from build123d import *

# Parameters (mm, degrees)
F1_DEPTH = 25
F2_R     = 2.296991
F2_R_2   = 2.582396
F3_DEPTH = 25
F5_DEPTH = 25


with BuildPart() as f1:
    # F0 (on Front) → F1 (new body)
    with BuildSketch(Plane.XZ):
        Polygon((0, 0), (0, 30), (-1.5, 30), (-1.5, 1.5), (-30, 1.5), (-30, 0), align=None)
    extrude(amount=F1_DEPTH)

    # F2 (on face) → F3 (cut)
    with BuildSketch(Plane.XY.offset(1.5)):
        with Locations((-22, -17)):
            Circle(F2_R)
        with Locations((-8, -8)):
            Circle(F2_R_2)
    extrude(amount=-F3_DEPTH, mode=Mode.SUBTRACT)

    # F4 (on face) → F5 (cut)
    with BuildSketch(Plane.YZ):
        with BuildLine():
            Line((-10.000746, 22.061086), (-10.00074, 21.93918))
            ThreePointArc((-10.00074, 21.93918), (-10, 22.000133), (-10.000746, 22.061086))
        make_face()
        with BuildLine():
            Line((-10, 8.000133), (-10.00074, 21.93918))
            Line((-10.00074, 21.93918), (-10.000746, 22.061086))
            ThreePointArc((-10.000746, 22.061086), (-12.495314, 24.499996), (-14.999007, 22.070455))
            Line((-14.999007, 22.070455), (-14.999007, 21.929545))
            Line((-14.999007, 21.929545), (-14.999007, 8.070455))
            Line((-14.999007, 8.070455), (-14.999007, 7.929545))
            ThreePointArc((-14.999007, 7.929545), (-12.464703, 5.500249), (-10, 8.000133))
        make_face()
        with BuildLine():
            Line((-14.999007, 21.929545), (-14.999007, 22.070455))
            ThreePointArc((-14.999007, 22.070455), (-15, 22), (-14.999007, 21.929545))
        make_face()
        with BuildLine():
            ThreePointArc((-14.999007, 8.070455), (-15, 8), (-14.999007, 7.929545))
            Line((-14.999007, 7.929545), (-14.999007, 8.070455))
        make_face()
    extrude(amount=-F5_DEPTH, mode=Mode.SUBTRACT)


solid = f1.part
Read the model definition and answer for the solid it produces. Units are mm, in the model's axes. A direction names the side the tool comes from. Round coordinates to 2 decimals unless told otherwise and drop trailing zeros. Write each loop counter-clockwise with the first axis right and the second up, starting at its lowest first coordinate (ties: lowest second). Pieces come first, ordered by that corner, then holes.
Q1. Find section A-A on x = -22. Determine the outline of the cut face in (y, z).
Values:
outline: (-25, 0) - (-19.3, 0) - (-19.3, 1.5) - (-25, 1.5) - close; (-14.7, 0) - (0, 0) - (0, 1.5) - (-14.7, 1.5) - close
Q2. Flat-ended cylindrical pins translate along their axes: P1, Ø12.5, axis at y = -11, z = 10, coming from the -X side; P2, Ø7.5, axis at x = -22, y = -17, coming from the +Z side. Find the tip coordinate at first contact, or state that the pin passes through.
Values:
P1: stops at x = -1.5
P2: stops at z = 1.5
Q3. Find section C-C on y = -18.5. Determine the outline of the cut face in (x, z).
Values:
outline: (-30, 0) - (-23.74, 0) - (-23.74, 1.5) - (-30, 1.5) - close; (-20.26, 0) - (0, 0) - (0, 30) - (-1.5, 30) - (-1.5, 1.5) - (-20.26, 1.5) - close
Q4. Find section D-D on y = -12.5. Determine the outline of the cut face in (x, z).
Values:
outline: (-30, 0) - (0, 0) - (0, 5.5) - (-1.5, 5.5) - (-1.5, 1.5) - (-30, 1.5) - close; (-1.5, 24.5) - (0, 24.5) - (0, 30) - (-1.5, 30) - close
Q5. Find section B-B on z = 6. Determine the outline of the cut face in (x, y), and give its area (3 significant figures).
Values:
outline: (-1.5, -25) - (0, -25) - (0, -14) - (-1.5, -14) - close; (-1.5, -11) - (0, -11) - (0, 0) - (-1.5, 0) - close
area: 33.0 mm2
Q6. The mould has two halves that part along Z. Classify faces 4 (the face through (-1, -12, 30)), 5 (the face through (-15, -12, 0)), 6 (the face through (-0.7, -12.4, 24.5)), 7 (the face through (-24.295, -16.899, 0.76)): released by +Z, released by -Z, zero draft, split by the parting line, or undercut.
Values:
face 4: released by +Z
face 5: released by -Z
face 6: undercut
face 7: zero draft
Q7. Straight lines are drawn through the part: line 1 (Y direction, x = -8, z = 0.6); line 2 (Y direction, x = -22, z = 0.7); line 3 (X direction, y = -19.5, z = 4.25). For each, find the intervals that lie inside material, in ascending order.
Values:
line 1: y = -25 to -10.58, -5.42 to 0
line 2: y = -25 to -19.3, -14.7 to 0
line 3: x = -1.5 to 0
Q8. A tool of negligible diameter and unlimited length cuts with its end or side. For faces 1 (the face through (0, -9.5, 14.8)), 2 (the face through (-1.5, -9.5, 15.9)), 3 (the face through (-1, -14.999, 15)), from which of +Z, -Z, +X, -X, +Y, -Y can it reach the whole face along a straight path? Write none if from no direction.
Values:
face 1: +Z, -Z, +X, +Y, -Y
face 2: +Z, -X, +Y, -Y
face 3: +X, -X
